from build123d import *

# Parameters (mm, degrees)
BOSS_EXTRUDE1_DEPTH = 24
SKETCH2_R           = 4
CUT_EXTRUDE1_DEPTH  = 30
SKETCH5_W           = 50
SKETCH5_H           = 40
SKETCH5_R           = 2.5
BOSS_EXTRUDE3_DEPTH = 4


with BuildPart() as part:
    # Sketch1 → Boss-Extrude1 (new, symmetric)
    with BuildSketch(Plane.XY):
        with BuildLine():
            Line((-22.873863542, 3), (-25, 3))
            Line((-25, 3), (-25, 12.5))
            Line((-25, 12.5), (25, 12.5))
            Line((25, 12.5), (25, -12.5))
            Line((25, -12.5), (-25, -12.5))
            Line((-25, -12.5), (-25, -3))
            Line((-25, -3), (-22.873863542, -3))
            ThreePointArc((-22.873863542, -3), (-8.5, 0), (-22.873863542, 3))
        make_face()
    extrude(amount=BOSS_EXTRUDE1_DEPTH, both=True)

    # Sketch2 → Cut-Extrude1 (cut)
    with BuildSketch(Plane(origin=(25, 0, 0), x_dir=(0, 0, -1), z_dir=(1, 0, 0))):
        with Locations((-15, 0)):
            Circle(SKETCH2_R)
        with Locations((15, 0)):
            Circle(SKETCH2_R)
    extrude(amount=-CUT_EXTRUDE1_DEPTH, mode=Mode.SUBTRACT)

    # Sketch5 → Boss-Extrude3 (add)
    with BuildSketch(Plane(origin=(0, 0, -24), x_dir=(-1, 0, 0), z_dir=(0, 0, -1))):
        with Locations((0, -32.5)):
            Rectangle(SKETCH5_W, SKETCH5_H)
        with Locations((0, -37.5)):
            Circle(SKETCH5_R, mode=Mode.SUBTRACT)
    extrude(amount=-BOSS_EXTRUDE3_DEPTH)


solid = part.part
Input: part model. Units: mm. Frame: model coordinates. A direction names the side the tool comes from. Coordinates: 2 decimals unless noted, no trailing zeros. Loops run counter-clockwise (first coordinate to the right, second up) from the corner with the lowest first, then second, coordinate; pieces in that order, holes last.
(1) Section C-C on x = -16. Return the cut outline in (y, z).
(2) Pull-direction query (Y, two-part tool) for faces 4 (the face through (-25, -11, -5)), 5 (the face through (0, -12.5, 2)), 6 (the face through (-24, -3, 0)); classes: released by +Y, released by -Y, zero draft, split by the parting line, or undercut.
(3) Section A-A on x = 0. Return the cut outline in (y, z).
(4) First-contact query: pin 1 Ø5 at (y, z) = (0, 15) entering from -X; pin 2 Ø10 at (x, y) = (17, -18) entering from +Z; pin 3 Ø1.5 at (x, z) = (1, 2) entering from -Y; pin 4 Ø3 at (x, y) = (0, -37.5) entering from -Z. Flat tips, straight axial feed; report the tip coordinate or a pass-through.
(5) Section B-B on y = -37.5. Return the cut outline in (x, z).
(6) Section D-D on z = 15. Return the cut outline in (x, y), then the cut area to 3 significant figures.
(7) Set-up query: faces 1 (the face through (0, -32, -20)), 2 (the face through (10, 0, -11)), 3 (the face through (-24, 3, 0)). Return all of +Z, -Z, +X, -X, +Y, -Y with unobstructed straight access to the full face (end or side cutting, diameter ignored); none if empty.
(8) Material intervals for probe 1 along Y at (x, z) = (12, -15); probe 2 along Y at (x, z) = (0, -22); probe 3 along Y at (x, z) = (-3.5, 3.5), sorted ascending.
Data:
1. outline: (-52.5, -24) - (-7.5, -24) - (-7.5, 24) - (-12.5, 24) - (-12.5, -20) - (-52.5, -20) - close; (7.5, -24) - (12.5, -24) - (12.5, 24) - (7.5, 24) - close
2. face 4: zero draft
2. face 5: released by -Y
2. face 6: undercut
3. outline: (-52.5, -24) - (-40, -24) - (-40, -20) - (-52.5, -20) - close; (-35, -24) - (12.5, -24) - (12.5, 24) - (-12.5, 24) - (-12.5, -20) - (-35, -20) - close; hole circle Ø8 at (0, -15); hole circle Ø8 at (0, 15)
4. pin 1: stops at x = -8.93
4. pin 2: stops at z = -20
4. pin 3: stops at y = -12.5
4. pin 4: passes through
5. outline: (-25, -24) - (-2.5, -24) - (-2.5, -20) - (-25, -20) - close; (2.5, -24) - (25, -24) - (25, -20) - (2.5, -20) - close
6. outline: (-25, -12.5) - (25, -12.5) - (25, -4) - (-5, -4) - (-5, 4) - (25, 4) - (25, 12.5) - (-25, 12.5) - (-25, 3) - (-22.87, 3) arc R7.5 cw (long way) to (-22.87, -3) - (-25, -3) - close
6. area: 823 mm2
7. face 1: +Z, +X, -X, -Y
7. face 2: +X
7. face 3: +Z, -Z, -X
8. probe 1: y = -12.5 to -4, 4 to 12.5
8. probe 2: y = -52.5 to -40, -35 to 12.5
8. probe 3: y = -12.5 to 12.5
